Can you work these out from the model? Positions are in its coordinate system, mm. Face numbers are marked on the shaded views. A direction names the side the tool comes from. Give positions to 0.01 mm unless a question says otherwise; leave off trailing zeros. Loops run counter-clockwise (first coordinate to the right, second up) from the corner with the lowest first, then second, coordinate; pieces in that order, holes last. Notation, with made-up numbers: (25.5, -13.75) -> (75.5, -13.75) arc R31 cw to (75.5, 22.25) -> close; hole circle Ø4 at (-17, 82). An arc over 180 degrees is marked (long way). Return JSON: item names as keys, results as strings. Group by question number.
Q1. Suppose I cut it at D-D, the plane x = 5.25. Please give me the cut outline in (y, z).
Q2. Suppose I cut it at C-C, the plane y = 1.2. Please give me the cut outline in (x, z), and give its area (3 significant figures).
Q3. I need wall thicknesses on line 1 along Z through (x, y) = (7, -1); line 2 along Y through (x, z) = (0.75, -5.75); line 3 along Z through (x, y) = (3.5, 0.7). Which ranges of each line are inside material? Lowest first, please. Write a range as [from, to].
Q4. Will these pins go through, and if not, where does the flat tip stop? pin 1 (1.5 mm diameter, centred on x = 6, z = -5.5, fed in from -Y); pin 2 (2 mm diameter, centred on y = -0.5, z = -2.5, fed in from +X); pin 3 (1.8 mm diameter, centred on x = 4.5, z = -4, fed in from -Y).
Q5. Suppose I cut it at B-B, the plane z = -3.75. Please give me the cut outline in (x, y), and give its area (3 significant figures).
Q6. Suppose I cut it at A-A, the plane x = 4. Please give me the cut outline in (y, z), and give its area (3 significant figures).
Q7. Thinking about a two-plate mould opening in X: for the marked faces 1, 2 and 3, which applies, pulls with the +X half, pulls with the -X half, needs draft (parallel to the pull), parting line crosses it, or undercut?
Q8. Which directions (+Z, -Z, +X, -X, +Y, -Y) give clear straight access to the entire face, cutting with the end or side of a thin tool? Please do the marked faces 4, 5 and 6.
```python
from build123d import *

# Parameters (mm, degrees)
SKETCH1_W               = 8
SKETCH1_H               = 8
BOSS_EXTRUDE1_DEPTH     = 3
CUT_EXTRUDE1_DEPTH      = 12.704699911
CUT_EXTRUDE1_DEPTH_BACK = 12.704699911
CUT_EXTRUDE2_DEPTH      = 11
SKETCH4_R               = 1.8
CUT_EXTRUDE3_DEPTH      = 0.8
SKETCH5_W               = 8
SKETCH5_H               = 1
BOSS_EXTRUDE2_DEPTH     = 2
FILLET1_R               = 4
CUT_EXTRUDE4_DEPTH      = 0.4


with BuildPart() as part:
    # Sketch1 → Boss-Extrude1 (new body)
    with BuildSketch(Plane(origin=(0, 0, 0), x_dir=(1, 0, 0), z_dir=(0, 1, 0))):
        with Locations((4, 4)):
            Rectangle(SKETCH1_W, SKETCH1_H)
    extrude(amount=BOSS_EXTRUDE1_DEPTH)

    # Sketch2 → Cut-Extrude1 (cut, two sides: drawn at the far end of the back side and taken through both)
    with BuildSketch(Plane.XY.offset(-CUT_EXTRUDE1_DEPTH_BACK)):
        Polygon((0, 0), (0.6, 3), (0, 3), align=None)
        Polygon((8, 0), (7.4, 3), (8, 3), align=None)
    extrude(amount=CUT_EXTRUDE1_DEPTH + CUT_EXTRUDE1_DEPTH_BACK, mode=Mode.SUBTRACT)

    # Sketch3 → Cut-Extrude2 (cut)
    with BuildSketch(Plane(origin=(0, 0, 0), x_dir=(0, 0, -1), z_dir=(1, 0, 0))):
        Polygon((0, 0), (0.6, 3), (0, 3), align=None)
        Polygon((8, 3), (7.4, 3), (8, 0), align=None)
    extrude(amount=CUT_EXTRUDE2_DEPTH, mode=Mode.SUBTRACT)

    # Sketch4 → Cut-Extrude3 (cut)
    with BuildSketch(Plane.XZ):
        with Locations(Location((4, -3.75, 0), (0, 0, 270))):
            Circle(SKETCH4_R)
    extrude(amount=-CUT_EXTRUDE3_DEPTH, mode=Mode.SUBTRACT)

    # Sketch5 → Boss-Extrude2 (add)
    with BuildSketch(Plane.XZ):
        with Locations((4, -7.5)):
            Rectangle(SKETCH5_W, SKETCH5_H)
    extrude(amount=BOSS_EXTRUDE2_DEPTH)

    # Fillet1
    # the kernel refuses this fillet: 4 mm, written as the material it takes off along each edge
    with BuildSketch(Plane(origin=(8, -2, -16.660254038), x_dir=(0, 1, 0), z_dir=(0, 0, 1)), Plane(origin=(0, -2, 1.660254038), x_dir=(0, 1, 0), z_dir=(0, 0, -1))) as fillet1_piece_1:
        with BuildLine():
            CenterArc((4, 3.464101615), FILLET1_R, 180, 60)
            Line((0, 3.464101615), (-0.08, 3.464101615))
            Line((-0.08, 3.464101615), (-0.08, 0))
            Line((-0.08, 0), (0, -0.08))
            ThreePointArc((0, -0.08), (1, -0.08), (1.96, -0.069282032))
            Line((1.96, -0.069282032), (2, 0))
        make_face()
    extrude(amount=18.320508076, mode=Mode.SUBTRACT)

    # Sketch6 → Cut-Extrude4 (cut)
    with BuildSketch(Plane(origin=(0, 3, 0), x_dir=(1, 0, 0), z_dir=(0, 1, 0))):
        Polygon((2.598201218, 2.07225421), (2.598201218, 6.07225421), (3.367431987, 6.07225421), (3.367431987, 2.738920877), (5.418714038, 2.738920877), (5.418714038, 2.07225421), align=None)
    extrude(amount=-CUT_EXTRUDE4_DEPTH, mode=Mode.SUBTRACT)


solid = part.part
```
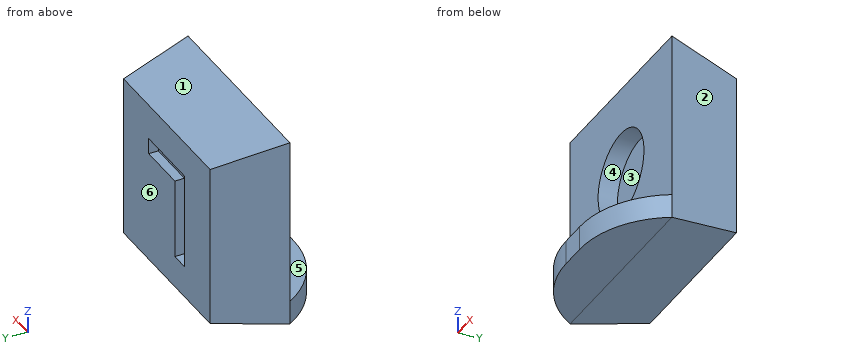
Ans:
{
 "1": {"outline": "(-1.94, -8) -> (0, -8) -> (3, -7.4) -> (3, -2.74) -> (2.6, -2.74) -> (2.6, -2.07) -> (3, -2.07) -> (3, -0.6) -> (0, 0) -> (0, -2.45) -> (0.8, -2.45) -> (0.8, -5.05) -> (0, -5.05) -> (0, -7) -> (-1.94, -7) -> close"},
 "2": {"outline": "(0.24, -7.76) -> (7.76, -7.76) -> (7.76, -0.24) -> (0.24, -0.24) -> close", "area": "56.6 mm^2"},
 "3": {"line 1": "z = [-8, -7]", "line 2": "y = [0, 3]", "line 3": "z = [-7.86, -5.48], [-2.02, -0.14]"},
 "4": {"pin 1": "stops at y = 0", "pin 2": "stops at x = 8", "pin 3": "stops at y = 0.8"},
 "5": {"outline": "(0, 0) -> (2.2, 0) -> (2.2, 0.8) -> (5.8, 0.8) -> (5.8, 0) -> (8, 0) -> (7.4, 3) -> (3.37, 3) -> (3.37, 2.6) -> (2.6, 2.6) -> (2.6, 3) -> (0.6, 3) -> close", "area": "19.0 mm^2"},
 "6": {"outline": "(-2, -8) -> (0, -8) -> (3, -7.4) -> (3, -2.74) -> (2.6, -2.74) -> (2.6, -2.07) -> (3, -2.07) -> (3, -0.6) -> (0, 0) -> (0, -1.95) -> (0.8, -1.95) -> (0.8, -5.55) -> (0, -5.55) -> (0, -7) -> (-2, -7) -> close", "area": "21.1 mm^2"},
 "7": {"face 1": "needs draft", "face 2": "pulls with the +X half", "face 3": "undercut"},
 "8": {"face 4": "-Y", "face 5": "+Z, +X, -X, -Y", "face 6": "+Z, -Z, +X, -X, +Y"}
}
